Can you work these out from the drawing? Everything is in mm from the part's minimum corner. A direction names the side the tool comes from. Give positions to 0.01 mm unless a question says otherwise; leave off trailing zeros. Loops run counter-clockwise (first coordinate to the right, second up) from the corner with the lowest first, then second, coordinate; pieces in that order, holes last.
Q1. Will these pins go through, and if not, where does the flat tip stop? P1, Ø1, axis at y = 55.5, z = 52.5, coming from the -X side; P2, Ø10, axis at y = 62.5, z = 13, coming from the +X side; P3, Ø6, axis at x = 112.5, y = 64.5, coming from the +Z side.
Q2. I need wall thicknesses on line 1 (Y direction, x = 185.5, z = 46); line 2 (X direction, y = 72.5, z = 33); line 3 (Z direction, x = 172, y = 70). Which ranges of each line are inside material? Lowest first, please.
Q3. If we section it at B-B (x = 155.5): Please give me the cut outline in (y, z), plus the area to 3 significant figures.
Q4. If we section it at A-A (z = 30): Please give me the cut outline in (x, y), plus the area to 3 significant figures.
Q5. If we section it at D-D (x = 209): Please give me the cut outline in (y, z), plus the area to 3 significant figures.
Q6. For the marked faces 1, 2 and 3, which set-ups out of +Z, -Z, +X, -X, +Y, -Y let a thin tool reach every point of the face, with its end or its side?
Q7. If we section it at C-C (z = 65): Please give me the cut outline in (x, y).
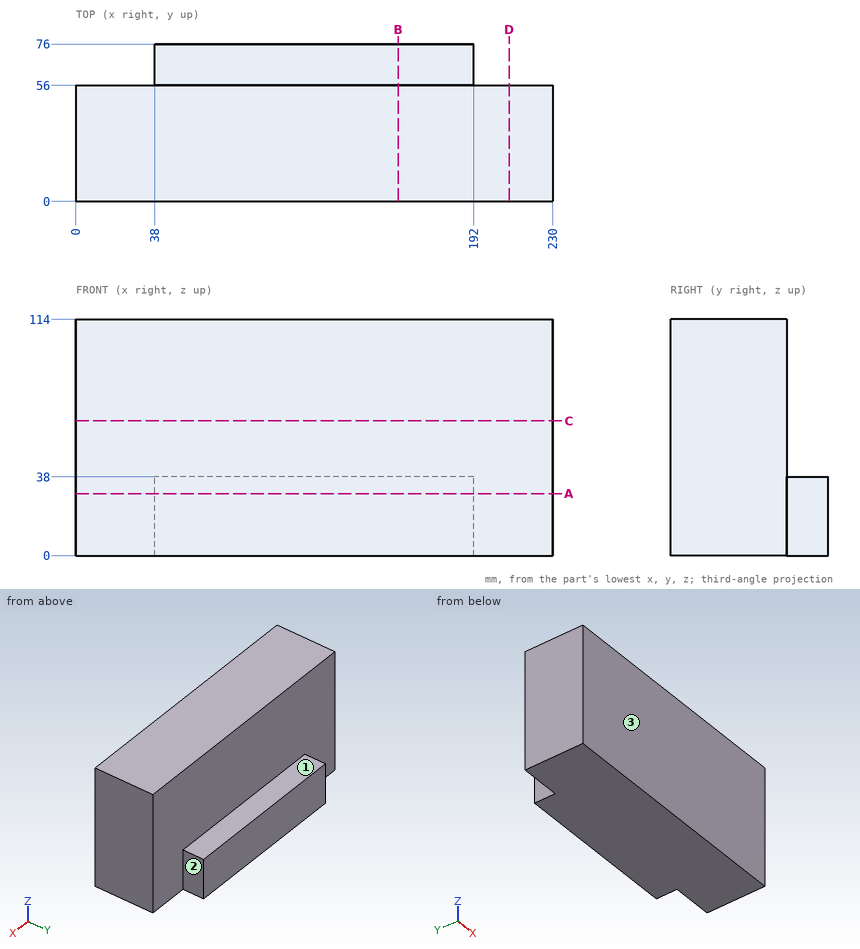
Check sheet entries:
1. P1: stops at x = 0
1. P2: stops at x = 192
1. P3: stops at z = 38
2. line 1: y = 0 to 56
2. line 2: x = 38 to 192
2. line 3: z = 0 to 38
3. outline: (0, 0) - (76, 0) - (76, 38) - (56, 38) - (56, 114) - (0, 114) - close
3. area: 7,140 mm2
4. outline: (0, 0) - (230, 0) - (230, 56) - (192, 56) - (192, 76) - (38, 76) - (38, 56) - (0, 56) - close
4. area: 16,000 mm2
5. outline: (0, 0) - (56, 0) - (56, 114) - (0, 114) - close
5. area: 6,380 mm2
6. face 1: +Z, +X, -X, +Y
6. face 2: +Z, -Z, +X, +Y
6. face 3: +Z, -Z, +X, -X, -Y
7. outline: (0, 0) - (230, 0) - (230, 56) - (0, 56) - close
